from build123d import *

# Parameters (mm, degrees)
F1_DEPTH  = 79.502
F2_W      = 30.8898873627
F2_H      = 37.5404208899
F3_DEPTH  = 25.4
F4_W      = 57.8284673393
F4_H      = 24.1576582193
F5_DEPTH  = 12.446
F6_W      = 72.3921172321
F6_H      = 23.4968811274
F7_DEPTH  = 21.082
F8_W      = 50.496625714
F8_H      = 17.7371860404
F9_DEPTH  = 56.388
F10_R     = 8.2310342768
F10_R_2   = 9.3664724304
F10_R_3   = 8.1183056078
F10_R_4   = 9.3356883849
F11_DEPTH = 85.344


with BuildPart() as f1:
    # F0 (on Front) → F1 (new body)
    with BuildSketch(Plane.XZ):
        Polygon((0, 37.5528037548), (-57.8284673393, 37.5528037548), (-57.8284673393, -13.5647049174), (0, -13.5647049174), (0, -23.8453224301), (61.8264861405, -23.8453224301), align=None)
    extrude(amount=F1_DEPTH)

    # F2 (on face) → F3 (cut)
    with BuildSketch(Plane.XY.offset(37.5528037548)):
        with Locations((-73.2734110206, -35.337369889)):
            Rectangle(F2_W, F2_H)
    extrude(amount=-F3_DEPTH, mode=Mode.SUBTRACT)

    # F4 (on face) → F5 (join)
    with BuildSketch(Plane.XY.offset(37.5528037548)):
        with Locations((-28.9142336696, -37.3493023217)):
            Rectangle(F4_W, F4_H)
    extrude(amount=-F5_DEPTH)

    # F6 (on face) → F7 (cut)
    with BuildSketch(Plane.XY.offset(37.5528037548)):
        with Locations((-21.6324087232, -34.1343507171)):
            Rectangle(F6_W, F6_H)
    extrude(amount=-F7_DEPTH, mode=Mode.SUBTRACT)

    # F8 (on face) → F9 (cut)
    with BuildSketch(Plane(origin=(0, 0, -23.8453224301), x_dir=(1, 0, 0), z_dir=(0, 0, -1))):
        with Locations((36.5781732835, 70.6334069798)):
            Rectangle(F8_W, F8_H)
    extrude(amount=-F9_DEPTH, mode=Mode.SUBTRACT)

    # F10 (on face) → F11 (cut)
    with BuildSketch(Plane(origin=(18.7759480822, 0, 18.9069433549), x_dir=(0.7095605761, 0, -0.7046444414), z_dir=(0.7046444414, 0, 0.7095605761))):
        with Locations((11.4842364565, -48.8504841924)):
            Circle(F10_R)
        with Locations((46.0814908147, -50.1335784793)):
            Circle(F10_R_2)
        with Locations((10.1835876703, -14.756876044)):
            Circle(F10_R_3)
        with Locations((44.260583818, -14.0236811712)):
            Circle(F10_R_4)
    extrude(amount=-F11_DEPTH, mode=Mode.SUBTRACT)


solid = f1.part
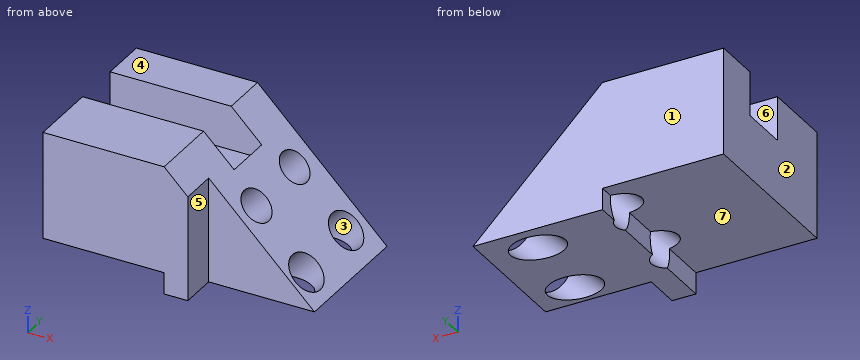
Verification items for the finished model (mm, model axes). Face numbers are marked on the shaded views. A direction names the side the tool comes from. Give positions to 0.01 mm unless a question says otherwise; leave off trailing zeros. Write each loop counter-clockwise with the first axis right and the second up, starting at its lowest first coordinate (ties: lowest second). Pieces come first, ordered by that corner, then holes.
(1) Gauge pin test, flat ends, axial feed: pin 1 (3 mm diameter, centred on x = -38.5, y = -43.5, fed in from -Z); pin 2 (3 mm diameter, centred on y = -39, z = 7, fed in from +X); pin 3 (14 mm diameter, centred on y = -71, z = -6, fed in from +X). Record the tip position at first contact, or that the pin passes through.
(2) Mould release check, pull along X, two halves, no side actions. Record for the marked faces 1, 2 and 3: +X half, -X half, draft (parallel to the pull), parting line (faces both ways), or undercut.
(3) Cross-section at D-D (z = 21). Enter the section's corners in (x, y), plus the area to 3 significant figures.
(4) Access from +Z, -Z, +X, -X, +Y, -Y to the whole of each face (thin tool, end or side, straight path). Record for the marked faces 4, 5, 6 and 7.
(5) Cross-section at A-A (y = -37). Enter the section's corners in (x, z).
(6) Cross-section at C-C (y = -52). Enter the section's corners in (x, z).
(7) Cross-section at B-B (x = -20). Enter the section's corners in (y, z), plus the area to 3 significant figures.
(8) Material ranges on line 1 (Y direction, x = 46.5, z = -17.5); line 2 (Y direction, x = -26.5, z = 24); line 3 (X direction, y = -63, z = 22.5), recorded low to high.
Worked out:
1. pin 1: stops at z = -13.56
1. pin 2: stops at x = 32.28
1. pin 3: stops at x = 11.33
2. face 1: draft
2. face 2: -X half
2. face 3: undercut
3. outline: (-57.83, -79.5) - (11.33, -79.5) - (11.33, -61.76) - (16.67, -61.76) - (16.67, 0) - (-57.83, 0) - (-57.83, -22.39) - (14.56, -22.39) - (14.56, -45.88) - (-57.83, -45.88) - close
3. area: 4,130 mm2
4. face 4: +Z, +X, -X, +Y, -Y
4. face 5: +Z, -Z, +X, -Y
4. face 6: +Z, -X
4. face 7: -Z, -X, +Y, -Y
5. outline: (-57.83, -13.56) - (0, -13.56) - (0, -23.85) - (61.83, -23.85) - (14.56, 23.09) - (14.56, 16.47) - (-57.83, 16.47) - close
6. outline: (-57.83, -13.56) - (-8, -13.56) - (21.53, 16.17) - (0, 37.55) - (-57.83, 37.55) - close; (3.22, -23.85) - (28.33, -23.85) - (44.96, -7.1) - (32.32, 5.46) - close; (54.2, -23.85) - (61.83, -23.85) - (57.99, -20.03) - close
7. outline: (-79.5, -13.56) - (0, -13.56) - (0, 37.55) - (-22.39, 37.55) - (-22.39, 16.47) - (-45.88, 16.47) - (-45.88, 37.55) - (-79.5, 37.55) - close
7. area: 3,570 mm2
8. line 1: y = -61.76 to -59.47, -40.8 to -23.3, -4.75 to 0
8. line 2: y = -79.5 to -45.88, -22.39 to 0
8. line 3: x = -57.83 to 11.33
